```python
from build123d import *

# Parameters (mm, degrees)
F1_DEPTH = 6.35
F3_D     = 8.7376
F5_DEPTH = 25.4
F6_R     = 12.7
F7_R     = 6.35


with BuildPart() as f1:
    # F0 (on Front) → F1 (new body)
    with BuildSketch(Plane.XZ):
        with BuildLine():
            Line((-141.7374620444, -81.8321618656), (-82.620901982, -47.7012))
            ThreePointArc((-82.620901982, -47.7012), (-75.6878127118, -58.0773013549), (-67.4596839815, -67.4596839815))
            Line((-67.4596839815, -67.4596839815), (-15.8232112853, -15.8232112853))
            ThreePointArc((-15.8232112853, -15.8232112853), (-20.6740218508, 8.5634602394), (0, 22.3774))
            Line((0, 22.3774), (0, 95.4024))
            ThreePointArc((0, 95.4024), (-71.1544614181, 63.5504566943), (-94.7963262761, -10.7365939814))
            Line((-94.7963262761, -10.7365939814), (-160.7874620444, -48.8365939814))
            Line((-160.7874620444, -48.8365939814), (-141.7374620444, -81.8321618656))
        make_face()
    extrude(amount=F1_DEPTH)

    # F3 (through all)
    with Locations(Plane.XZ.offset(6.35)):
        with Locations((-44.2468, 76.6377056723), (-76.6377056723, -44.2468)):
            Hole(F3_D / 2)

    # F4 (on face) → F5 (join)
    with BuildSketch(Plane.XZ.offset(6.35)):
        Polygon((-136.2382007304, -78.6571618656), (-155.2882007304, -45.6615939814), (-160.7874620444, -48.8365939814), (-141.7374620444, -81.8321618656), align=None)
    extrude(amount=F5_DEPTH)

    # F6
    f6_edges = [f1.edges().sort_by_distance(p)[0] for p in [
        (-82.620902, -3.175, -47.7012),
        (-94.796326, -3.175, -10.736594),
    ]]
    fillet(f6_edges, radius=F6_R)

    # F7
    f7_edges = [f1.edges().sort_by_distance(p)[0] for p in [
        (-67.459684, -3.175, -67.459684),
        (-15.823211, -3.175, -15.823211),
        (0, -3.175, 22.3774),
        (0, -3.175, 95.4024),
    ]]
    fillet(f7_edges, radius=F7_R)


solid = f1.part
```
Work out the finished part from the listing and answer in its coordinate system (mm). Round coordinates to 2 decimals unless told otherwise and drop trailing zeros. Loops run counter-clockwise (first coordinate to the right, second up) from the corner with the lowest first, then second, coordinate; pieces in that order, holes last. Notation, with made-up numbers: (76, -2) -> (133, -2) arc R10 ccw to (133, 16) -> close; hole circle Ø9 at (7, 88). An arc over 180 degrees is marked (long way). Write each question's results on one line, items separated by ' | '. Start each with the question number.
1. Section A-A (y = -17) is taken. Determine the outline of the cut face in (x, z).
2. Section C-C (z = 11.5) is taken. Determine the outline of the cut face in (x, y), plus the area to 3 significant figures.
3. Given pin 1 Ø10 at (x, y) = (-115, -13.5) entering from +Z; pin 2 Ø1 at (x, z) = (-53, 8) entering from -Y; pin 3 Ø8 at (y, z) = (-6.5, -60.5) entering from -X, each flat-ended and moving along its own axis, determine where each tip first touches the part or whether it passes through.
4. For a pull along X with two mould halves and no side action, classify faces 1 (the face through (-74.35, -3.13, -59.78)), 2 (the face through (-78.7, -3.1, -48.1)), 3 (the face through (-145.63, -18.87, -62.39)), 4 (the face through (-149, -31.75, -64)) as +X half, -X half, draft (parallel to the pull), parting line (faces both ways), or undercut.
5. Section B-B (x = -145.5) is taken. Determine the outline of the cut face in (y, z), plus the area to 3 significant figures.
6. Find the intervals of material crossed by probe 1 along Y at (x, z) = (-30, 18); probe 2 along X at (y, z) = (-5, 77.5), in increasing order. Write a range as from..to.
Evaluation:
1) outline: (-160.79, -48.84) -> (-141.74, -81.83) -> (-136.24, -78.66) -> (-155.29, -45.66) -> close
2) outline: (-94.71, -6.35) -> (-19.2, -6.35) -> (-19.2, 0) -> (-94.71, 0) -> close | area: 479 mm2
3) pin 1: passes through | pin 2: stops at y = -6.35 | pin 3: stops at x = -156.36
4) face 1: undercut | face 2: undercut | face 3: +X half | face 4: draft
5) outline: (-31.75, -75.32) -> (0, -75.32) -> (0, -40.01) -> (-6.35, -40.01) -> (-6.35, -62.62) -> (-31.75, -62.62) -> close | area: 547 mm2
6) probe 1: y = -6.35..0 | probe 2: x = -55.64..-48.53, -39.96..0
